from build123d import *

# Parameters (mm, degrees)
F1_DEPTH = 30


with BuildPart() as f1:
    # F0 (on Front) → F1 (new body, symmetric)
    with BuildSketch(Plane.XZ):
        Polygon((22.305341, 0), (0, 0), (-22.305341, 0), (-22.305341, -6.29586), (-41.732572, -6.29586), (-41.732572, -17.44853), (-25.543211, -17.44853), (-25.543211, -27.52191), (-12.951488, -27.52191), (-12.951488, -21.765692), (0, -21.765692), (12.951488, -21.765692), (12.951488, -27.52191), (25.543211, -27.52191), (25.543211, -17.44853), (41.732572, -17.44853), (41.732572, -6.29586), (22.305341, -6.29586), align=None)
    extrude(amount=F1_DEPTH, both=True)


solid = f1.part
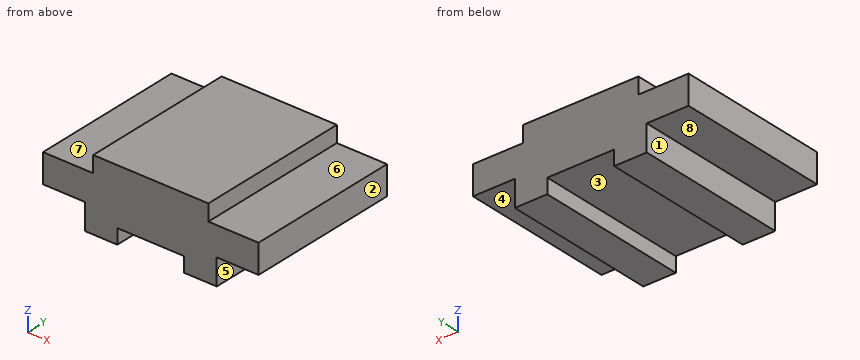
Check sheet for the modelled part. Datum: model origin and axes. Units: mm. Face numbers are marked on the shaded views. A direction names the side the tool comes from. Round coordinates to 2 decimals unless told otherwise and drop trailing zeros. Write each loop counter-clockwise with the first axis right and the second up, starting at its lowest first coordinate (ties: lowest second). Pieces come first, ordered by that corner, then holes. Notation, with made-up numbers: (5.25, -0.5) - (40.25, -0.5) arc R17 ccw to (40.25, 7.5) - close; hole circle Ø3 at (-26.75, 30). An arc over 180 degrees is marked (long way). Return JSON: item names as keys, results as strings.
Q1. Cross-section at D-D (z = -19). Record the boundary of the cut face in (x, y).
Returned:
{"outline": "(-25.54, -30) - (25.54, -30) - (25.54, 30) - (-25.54, 30) - close"}
Q2. Cross-section at A-A (z = -25.5). Record the boundary of the cut face in (x, y).
Returned:
{"outline": "(-25.54, -30) - (-12.95, -30) - (-12.95, 30) - (-25.54, 30) - close; (12.95, -30) - (25.54, -30) - (25.54, 30) - (12.95, 30) - close"}
Q3. Cross-section at B-B (y = -15.5). Record the boundary of the cut face in (x, z), then the cut area to 3 significant figures.
Returned:
{"outline": "(-41.73, -17.45) - (-25.54, -17.45) - (-25.54, -27.52) - (-12.95, -27.52) - (-12.95, -21.77) - (12.95, -21.77) - (12.95, -27.52) - (25.54, -27.52) - (25.54, -17.45) - (41.73, -17.45) - (41.73, -6.3) - (22.31, -6.3) - (22.31, 0) - (-22.31, 0) - (-22.31, -6.3) - (-41.73, -6.3) - close", "area": "1,580 mm²"}
Q4. Cross-section at C-C (x = 4.5). Record the boundary of the cut face in (y, z), then the cut area to 3 significant figures.
Returned:
{"outline": "(-30, -21.77) - (30, -21.77) - (30, 0) - (-30, 0) - close", "area": "1,310 mm²"}
Q5. Scan lines: L1, parallel to X at y = 21.5, z = -26; L2, parallel to X at y = -12, z = -3.25; L3, parallel to Z at x = -27.5, y = -5.5. Record each from-to range of solid material in increasing order. Write a range as from..to.
Returned:
{"L1": "x = -25.54..-12.95, 12.95..25.54", "L2": "x = -22.31..22.31", "L3": "z = -17.45..-6.3"}
Q6. Access from +Z, -Z, +X, -X, +Y, -Y to the whole of each face (thin tool, end or side, straight path). Record for the marked faces 5, 6, 7 and 8.
Returned:
{"face 5": "-Z, +X, +Y, -Y", "face 6": "+Z, +X, +Y, -Y", "face 7": "+Z, -X, +Y, -Y", "face 8": "-Z, -X, +Y, -Y"}
Q7. Depth check by flat-ended pin: P1, Ø20.5, axis at x = 3, y = 8.5, coming from the -Z side; P2, Ø21.5, axis at x = 37, y = -2, coming from the +Z side; P3, Ø1.9, axis at y = 10, z = -1.5, coming from the -X side; P4, Ø6, axis at y = 22, z = -21.5, coming from the -X side. Enter the tip coordinate at first touch or a pass-through.
Returned:
{"P1": "stops at z = -27.52", "P2": "stops at z = -6.3", "P3": "stops at x = -22.31", "P4": "stops at x = -25.54"}
Q8. Draft check along X on the marked faces 1, 2, 3 and 4. Enter one of: released by +X, released by -X, zero draft, split by the parting line, or undercut.
Returned:
{"face 1": "released by -X", "face 2": "released by +X", "face 3": "undercut", "face 4": "zero draft"}
